Verification items for the finished model (mm, model axes). Face numbers are marked on the shaded views. A direction names the side the tool comes from. Give positions to 0.01 mm unless a question says otherwise; leave off trailing zeros. Loops run counter-clockwise (first coordinate to the right, second up) from the corner with the lowest first, then second, coordinate; pieces in that order, holes last. Notation, with made-up numbers: (59, 25.5) - (117, 25.5) arc R7 cw to (117, 38.5) - close; hole circle Ø2 at (48, -13). An arc over 180 degrees is marked (long way). Answer in a Markdown table with one row per item.
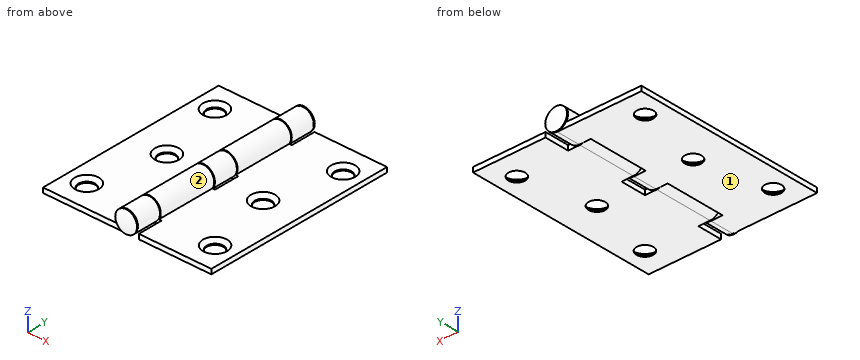
```python
from build123d import *

# Parameters (mm, degrees)
BOSS_EXTRUDE1_START          = -4.318
SKETCH3_W                    = 33.3375
SKETCH3_H                    = 76.2
SKETCH3_R                    = 3.302
BOSS_EXTRUDE1_DEPTH          = 1.905
CUT_EXTRUDE_THIN1_DEPTH      = 51.661898224
CUT_EXTRUDE_THIN1_DEPTH_BACK = 51.661898224
CUT_EXTRUDE2_DEPTH           = 51.661898224
CUT_EXTRUDE2_DEPTH_BACK      = 51.661898224
SKETCH6_W                    = 33.3375
SKETCH6_H                    = 76.2
CUT_EXTRUDE3_DEPTH           = 51.661898224
CUT_EXTRUDE3_DEPTH_BACK      = 51.661898224
SKETCH7_W                    = 33.3375
SKETCH7_H                    = 76.2
SKETCH8_R                    = 4.318
BOSS_EXTRUDE2_DEPTH          = 9.525
SKETCH9_R                    = 4.318
BOSS_EXTRUDE3_DEPTH          = 9.525
SKETCH10_R                   = 4.318
BOSS_EXTRUDE4_DEPTH          = 9.525
SKETCH11_R                   = 4.318
BOSS_EXTRUDE5_DEPTH          = 23.1775
SKETCH12_R                   = 4.318
BOSS_EXTRUDE6_DEPTH          = 23.1775
BOSS_EXTRUDE8_START          = 0.127
SKETCH15_R                   = 4.318
BOSS_EXTRUDE8_DEPTH          = 0.3175
DOME1_FACE_RADIUS            = 4.318
DOME1_HEIGHT                 = 1.27
BOSS_EXTRUDE7_START          = -38.227
SKETCH13_R                   = 2.38125
BOSS_EXTRUDE7_DEPTH          = 76.454


with BuildPart() as part:
    # Sketch3 → Boss-Extrude1 (new body)
    with BuildSketch(Plane.XY.offset(BOSS_EXTRUDE1_START)):
        with Locations((-16.66875, 0)):
            Rectangle(SKETCH3_W, SKETCH3_H)
        with Locations((-25.4, 27.78125)):
            Circle(SKETCH3_R, mode=Mode.SUBTRACT)
        with Locations((-19.05, 0)):
            Circle(SKETCH3_R, mode=Mode.SUBTRACT)
        with Locations((-25.4, -27.78125)):
            Circle(SKETCH3_R, mode=Mode.SUBTRACT)
    extrude(amount=BOSS_EXTRUDE1_DEPTH)

    # Cut-Extrude1 cone 1 section (through the dimple's axis) → Cut-Extrude1 (revolve, cut)
    with BuildSketch(Plane(origin=(-25.4, 27.78125, -2.413), x_dir=(0, -1, 0), z_dir=(1, 0, 0))):
        Polygon((0, 0), (4.7625, 0), (0, 4.7625), align=None)
    revolve(axis=Axis((-25.4, 27.78125, -2.413), (0, 0, -1)), mode=Mode.SUBTRACT)

    # Cut-Extrude1 cone 2 section (through the dimple's axis) → Cut-Extrude1 cone 2 (revolve, cut)
    with BuildSketch(Plane(origin=(-19.05, 0, -2.413), x_dir=(0, -1, 0), z_dir=(1, 0, 0))):
        Polygon((0, 0), (4.7625, 0), (0, 4.7625), align=None)
    revolve(axis=Axis((-19.05, 0, -2.413), (0, 0, -1)), mode=Mode.SUBTRACT)

    # Cut-Extrude1 cone 3 section (through the dimple's axis) → Cut-Extrude1 cone 3 (revolve, cut)
    with BuildSketch(Plane(origin=(-25.4, -27.78125, -2.413), x_dir=(0, -1, 0), z_dir=(1, 0, 0))):
        Polygon((0, 0), (4.7625, 0), (0, 4.7625), align=None)
    revolve(axis=Axis((-25.4, -27.78125, -2.413), (0, 0, -1)), mode=Mode.SUBTRACT)

    # Mirror1: part across plane


with BuildPart() as part_1:
    add(part.part)
    add(part.part.mirror(Plane(origin=(0, 0, 0), x_dir=(0, 0, 1), z_dir=(1, 0, 0))))

    # Sketch5 → Cut-Extrude-Thin1 (cut, two sides: drawn at the far end of the back side and taken through both)
    with BuildSketch(Plane.XY.offset(-2.413).offset(-CUT_EXTRUDE_THIN1_DEPTH_BACK)):
        Polygon((4.318, 38.1), (4.318, 28.575), (-4.6355, 28.575), (-4.6355, 4.7625), (4.318, 4.7625), (4.318, 0), (4.318, -4.7625), (-4.6355, -4.7625), (-4.6355, -28.575), (4.318, -28.575), (4.318, -38.1), (4.6355, -38.1), (4.6355, -28.2575), (-4.318, -28.2575), (-4.318, -5.08), (4.6355, -5.08), (4.6355, 0), (4.6355, 5.08), (-4.318, 5.08), (-4.318, 28.2575), (4.6355, 28.2575), (4.6355, 38.1), align=None)
    extrude(amount=CUT_EXTRUDE_THIN1_DEPTH + CUT_EXTRUDE_THIN1_DEPTH_BACK, mode=Mode.SUBTRACT)


with BuildPart() as cut_extrude_thin1_piece_1:
    # of the separate pieces the step leaves, piece 1, a body of its own (cut_extrude_thin1_pieces)
    add(part_1.part.solids().sort_by_distance((4.6355, 38.1, -4.318))[0])

    # Sketch6 → Cut-Extrude2 (cut, two sides: drawn at the far end of the back side and taken through both)
    with BuildSketch(Plane.XY.offset(-2.413).offset(-CUT_EXTRUDE2_DEPTH_BACK)):
        with Locations((-16.66875, 0)):
            Rectangle(SKETCH6_W, SKETCH6_H)
    extrude(amount=CUT_EXTRUDE2_DEPTH + CUT_EXTRUDE2_DEPTH_BACK, mode=Mode.SUBTRACT)

    # Sketch11 → Boss-Extrude5 (add)
    with BuildSketch(Plane.XZ.offset(28.2575)):
        Circle(SKETCH11_R)
    extrude(amount=-BOSS_EXTRUDE5_DEPTH)

    # Sketch12 → Boss-Extrude6 (add)
    with BuildSketch(Plane(origin=(0, 28.2575, 0), x_dir=(1, 0, 0), z_dir=(0, 1, 0))):
        Circle(SKETCH12_R)
    extrude(amount=-BOSS_EXTRUDE6_DEPTH)



with BuildPart() as cut_extrude_thin1_piece_2:
    # of the separate pieces the step leaves, piece 2, a body of its own (cut_extrude_thin1_pieces)
    add(part_1.part.solids().sort_by_distance((-33.3375, 38.1, -4.318))[0])

    # Sketch7 → Cut-Extrude3 (cut, two sides: drawn at the far end of the back side and taken through both)
    with BuildSketch(Plane.XY.offset(-2.413).offset(-CUT_EXTRUDE3_DEPTH_BACK)):
        with Locations((16.66875, 0)):
            Rectangle(SKETCH7_W, SKETCH7_H)
    extrude(amount=CUT_EXTRUDE3_DEPTH + CUT_EXTRUDE3_DEPTH_BACK, mode=Mode.SUBTRACT)

    # Sketch8 → Boss-Extrude2 (add)
    with BuildSketch(Plane.XZ.offset(38.1)):
        Circle(SKETCH8_R)
    extrude(amount=-BOSS_EXTRUDE2_DEPTH)

    # Sketch9 → Boss-Extrude3 (add)
    with BuildSketch(Plane.XZ.offset(4.7625)):
        Circle(SKETCH9_R)
    extrude(amount=-BOSS_EXTRUDE3_DEPTH)

    # Sketch10 → Boss-Extrude4 (add)
    with BuildSketch(Plane.XZ.offset(-28.575)):
        Circle(SKETCH10_R)
    extrude(amount=-BOSS_EXTRUDE4_DEPTH)


with BuildPart() as body_3:
    # Sketch15 → Boss-Extrude8 (new body)
    with BuildSketch(Plane(origin=(0, 38.1, 0), x_dir=(1, 0, 0), z_dir=(0, 1, 0)).offset(BOSS_EXTRUDE8_START)):
        with Locations(Location((0, 0, 0), (0, 0, 270))):
            Circle(SKETCH15_R)
    extrude(amount=BOSS_EXTRUDE8_DEPTH)

    # Dome1: a dome of height H over a round flat face of radius A is a cap of a sphere of radius (A * A + H * H) / (2 * H)
    dome1_r = (DOME1_FACE_RADIUS * DOME1_FACE_RADIUS + DOME1_HEIGHT * DOME1_HEIGHT) / (2 * DOME1_HEIGHT)
    dome1_base = Plane((0, 38.5445, 0), z_dir=(0, 1, 0))
    with Locations(dome1_base.offset(DOME1_HEIGHT - dome1_r)):
        dome1_ball = Sphere(dome1_r, mode=Mode.PRIVATE)
    add(split(dome1_ball, bisect_by=dome1_base, keep=Keep.TOP, mode=Mode.PRIVATE))


with BuildPart() as body_4:
    # Mirror2: mirrored copy
    add(body_3.part.mirror(Plane.ZX))


with BuildPart() as cut_extrude_thin1_piece_1_1:
    add(cut_extrude_thin1_piece_1.part)

    add(cut_extrude_thin1_piece_2.part)  # Boss-Extrude7 merges Cut-Extrude-Thin1 piece 2

    add(body_3.part)  # Boss-Extrude7 merges body 3

    add(body_4.part)  # Boss-Extrude7 merges body 4
    # Sketch13 → Boss-Extrude7 (add)
    with BuildSketch(Plane(origin=(0, 0, 0), x_dir=(1, 0, 0), z_dir=(0, 1, 0)).offset(BOSS_EXTRUDE7_START)):
        with Locations(Location((0, 0, 0), (0, 0, 270))):
            Circle(SKETCH13_R)
    extrude(amount=BOSS_EXTRUDE7_DEPTH)


solid = cut_extrude_thin1_piece_1_1.part
```
Q1. Sectioned sample at A-A (y = 0). Record the cut outline in (x, z), and give its area (3 significant figures).
Completed:
| item | result |
|---|---|
| outline | (-33.34, -4.32) - (-22.35, -4.32) - (-22.35, -3.87) - (-23.81, -2.41) - (-33.34, -2.41) - close; (-15.75, -4.32) - (0, -4.32) arc R4.32 ccw (long way) to (-3.58, -2.41) - (-14.29, -2.41) - (-15.75, -3.87) - close; (4.64, -4.32) - (15.75, -4.32) - (15.75, -3.87) - (14.29, -2.41) - (4.64, -2.41) - close; (22.35, -4.32) - (33.34, -4.32) - (33.34, -2.41) - (23.81, -2.41) - (22.35, -3.87) - close |
| area | 143 mm^2 |
Q2. Tool access check on the marked faces 1 and 2. Record the directions out of +Z, -Z, +X, -X, +Y, -Y that give a thin tool (end or side, any length) a straight path to the whole face; none if there is none.
Completed:
| item | result |
|---|---|
| face 1 | -Z, +X, -X, +Y, -Y |
| face 2 | none |
Q3. Go/stop test with flat-tipped pins: P1, Ø1.5, axis at x = 21, z = -3.5, coming from the +Y side; P2, Ø2.5, axis at x = 2, z = 0, coming from the +Y side; P3, Ø3, axis at x = -15.5, z = -2, coming from the -Y side; P4, Ø7.5, axis at x = -25.4, y = -27.78, coming from the -Z side. Record where each tip stops, or that it passes through.
Completed:
| item | result |
|---|---|
| P1 | y = 38.1 |
| P2 | y = 39.78 |
| P3 | y = -38.1 |
| P4 | z = -4.32 |
Q4. Sectioned sample at B-B (x = -25.4). Record the cut outline in (y, z).
Completed:
| item | result |
|---|---|
| outline | (-38.1, -4.32) - (-31.08, -4.32) - (-31.08, -3.87) - (-32.54, -2.41) - (-38.1, -2.41) - close; (-24.48, -4.32) - (24.48, -4.32) - (24.48, -3.87) - (23.02, -2.41) - (-23.02, -2.41) - (-24.48, -3.87) - close; (31.08, -4.32) - (38.1, -4.32) - (38.1, -2.41) - (32.54, -2.41) - (31.08, -3.87) - close |
Q5. Thickness scan on line 1 (Y direction, x = -25.4, z = -4.1); line 2 (Y direction, x = 11, z = -2.5); line 3 (X direction, y = -20.5, z = -0.25). Record the ranges inside material, lowest first.
Completed:
| item | result |
|---|---|
| line 1 | -38.1 to -31.08, -24.48 to 24.48, 31.08 to 38.1 |
| line 2 | -38.1 to 38.1 |
| line 3 | -4.31 to 4.31 |
